```python
from build123d import *

# Parameters (mm, degrees)
SKETCH1_W           = 203.2
SKETCH1_H           = 101.6
SKETCH1_W_2         = 165.1
SKETCH1_H_2         = 63.5
BOSS_EXTRUDE1_DEPTH = 50.8
SKETCH2_R           = 7.9375
CUT_EXTRUDE1_DEPTH  = 50.8


with BuildPart() as part:
    # Sketch1 → Boss-Extrude1 (new body)
    with BuildSketch(Plane.XY):
        with Locations((101.6, 50.8)):
            Rectangle(SKETCH1_W, SKETCH1_H)
        with Locations((101.6, 50.8)):
            Rectangle(SKETCH1_W_2, SKETCH1_H_2, mode=Mode.SUBTRACT)
    extrude(amount=BOSS_EXTRUDE1_DEPTH)

    # Sketch2 → Cut-Extrude1 (cut)
    with BuildSketch(Plane.ZY):
        with Locations((25.4, 50.8)):
            Circle(SKETCH2_R)
    extrude(amount=-CUT_EXTRUDE1_DEPTH, mode=Mode.SUBTRACT)


solid = part.part
```
Check sheet for the modelled part. Datum: model origin and axes. Units: mm. A direction names the side the tool comes from. Round coordinates to 2 decimals unless told otherwise and drop trailing zeros. Loops run counter-clockwise (first coordinate to the right, second up) from the corner with the lowest first, then second, coordinate; pieces in that order, holes last. Notation, with made-up numbers: M 36.5,7.5 L 54.5,7.5 A22 cw 54.5,24.5 Z; hole C 18,53 d1. An arc over 180 degrees is marked long. Answer as a JSON object with one key per item and string values.
1. Section check C-C (y = 36). Record the boundary of the cut face in (x, z).
Reply:
{"outline": "M 0,0 L 19.05,0 L 19.05,50.8 L 0,50.8 Z; M 184.15,0 L 203.2,0 L 203.2,50.8 L 184.15,50.8 Z"}
2. Access from +Z, -Z, +X, -X, +Y, -Y to the whole of each face (thin tool, end or side, straight path). Record for faces 1 (the cylindrical face through (9.392, 56.165, 19.55)), 2 (the flat face through (19.05, 43, 31)), 3 (the flat face through (100, 85, 50.8)).
Reply:
{"face 1": "-X", "face 2": "+Z, -Z", "face 3": "+Z, +X, -X, +Y, -Y"}
3. Scan lines: line 1 (Y direction, x = 4.25, z = 25.4); line 2 (Y direction, x = 60.5, z = 33.5); line 3 (X direction, y = 80, z = 43). Record each from-to range of solid material in increasing order.
Reply:
{"line 1": "y = 0 to 42.86, 58.74 to 101.6", "line 2": "y = 0 to 19.05, 82.55 to 101.6", "line 3": "x = 0 to 19.05, 184.15 to 203.2"}
4. Section check A-A (y = 50.8). Record the boundary of the cut face in (x, z), plus the area to 3 significant figures.
Reply:
{"outline": "M 0,0 L 19.05,0 L 19.05,17.46 L 0,17.46 Z; M 0,33.34 L 19.05,33.34 L 19.05,50.8 L 0,50.8 Z; M 184.15,0 L 203.2,0 L 203.2,50.8 L 184.15,50.8 Z", "area": "1,630 mm²"}
5. Section check D-D (z = 25.4). Record the boundary of the cut face in (x, y), plus the area to 3 significant figures.
Reply:
{"outline": "M 0,0 L 203.2,0 L 203.2,101.6 L 0,101.6 L 0,58.74 L 19.05,58.74 L 19.05,82.55 L 184.15,82.55 L 184.15,19.05 L 19.05,19.05 L 19.05,42.86 L 0,42.86 Z", "area": "9,860 mm²"}
6. Section check B-B (x = 29). Record the boundary of the cut face in (y, z), plus the area to 3 significant figures.
Reply:
{"outline": "M 0,0 L 19.05,0 L 19.05,50.8 L 0,50.8 Z; M 82.55,0 L 101.6,0 L 101.6,50.8 L 82.55,50.8 Z", "area": "1,940 mm²"}
7. Mould release check, pull along X, two halves, no side actions. Record for faces 4 (the flat face through (0, 61, 25)), 5 (the flat face through (100, 19.05, 25)), 6 (the flat face through (184.15, 50, 25)), 7 (the flat face through (100, 0, 25)): pulls with the +X half, pulls with the -X half, needs draft (parallel to the pull), parting line crosses it, or undercut.
Reply:
{"face 4": "pulls with the -X half", "face 5": "undercut", "face 6": "undercut", "face 7": "needs draft"}
8. Gauge pin test, flat end, axial feed: P1, Ø10, axis at y = 21.5, z = 17.5, coming from the -X side. Record the tip position at first contact, or that the pin passes through.
Reply:
{"P1": "stops at x = 0"}
